```python
from build123d import *


with BuildPart() as f1:
    # F0 (on Top) → F1 (revolve)
    with BuildSketch(Plane.XY):
        with BuildLine():
            Line((5, -24.18787), (5, -20.135133))
            Line((5, -20.135133), (5, -17.787319))
            Line((5, -17.787319), (13, -17.787319))
            Line((13, -17.787319), (25.4, -9.104746))
            Line((25.4, -9.104746), (25.4, 13.497188))
            ThreePointArc((25.4, 13.497188), (24.003098, 16.599398), (20.846833, 17.869453))
            Line((20.846833, 17.869453), (0, 17.869453))
            Line((0, 17.869453), (-20.847, 17.869453))
            ThreePointArc((-20.847, 17.869453), (-24.003206, 16.599388), (-25.4, 13.497184))
            Line((-25.4, 13.497184), (-25.4, -9.104746))
            Line((-25.4, -9.104746), (-13, -17.787319))
            Line((-13, -17.787319), (-5, -17.787319))
            Line((-5, -17.787319), (-5, -20.135133))
            Line((-5, -20.135133), (-5, -24.18787))
            Line((-5, -24.18787), (5, -24.18787))
        make_face()
    revolve(axis=Axis((1.997764, -32.846637, 0), (1, 0, 0)))

    # F2: F1 across plane


with BuildPart() as f1_1:
    add(f1.part)
    add(f1.part.mirror(Plane.XY))


solid = f1_1.part
```
Work out the finished part from the listing and answer in its coordinate system (mm). A direction names the side the tool comes from. Give positions to 0.01 mm unless a question says otherwise; leave off trailing zeros. Loops run counter-clockwise (first coordinate to the right, second up) from the corner with the lowest first, then second, coordinate; pieces in that order, holes last. Notation, with made-up numbers: M 61,19.25 L 76,19.25 A24 ccw 76,48.25 Z; hole C 12.5,21.5 d6. An arc over 180 degrees is marked long. One line per item, written item: value. Start each with the question number.
1. Find section A-A (z = 0). Give the vertices of the cut face in (x, y).
2. Determine the mould class of faces 1 (the face through (-0.292, -39.449, 50.285)), 2 (the face through (-8.944, -18.936, -5.768)), 3 (the face through (-25.4, -54.09, 10.95)) for opening direction Y: released by +Y, released by -Y, zero draft, split by the parting line, or undercut.
3. Which of the six approach directions +Z, -Z, +X, -X, +Y, -Y give full straight-line access (tool end or side, diameter ignored) to faces 4 (the face through (9.056, -18.936, -5.768)), 5 (the face through (25.4, -11.6, 10.95)), 6 (the face through (-5, -26, -6))?
4. Find the intervals of material crossed by probe 1 along X at (y, z) = (-58, 39); probe 2 along Z at (x, y) = (-22, -21); probe 3 along Z at (x, y) = (16.5, -31), in increasing order.
5. Each of these flat-tipped pins is pushed along its axis until it touches: P1, Ø24, axis at y = -31, z = 0.5, coming from the +X side; P2, Ø12, axis at x = -6.5, z = -35, coming from the +Y side; P3, Ø4, axis at x = -6.5, y = -52, coming from the -Z side. Where does it stop, or does it pass through?
6. Find section C-C (x = 15). Give the vertices of the cut face in (y, z).
7. Find section B-B (x = 6.5). Give the vertices of the cut face in (y, z), and give its area (3 significant figures).
Reported:
1. outline: M -25.4,-79.19 A4.56 ccw -20.85,-83.56 L 20.85,-83.56 A4.56 ccw 25.4,-79.19 L 25.4,-56.59 L 13,-47.91 L 5,-47.91 L 5,-41.51 L -5,-41.51 L -5,-47.91 L -13,-47.91 L -25.4,-56.59 Z; M -25.4,-9.1 L -13,-17.79 L -5,-17.79 L -5,-24.19 L 5,-24.19 L 5,-17.79 L 13,-17.79 L 25.4,-9.1 L 25.4,13.5 A4.56 ccw 20.85,17.87 L -20.85,17.87 A4.56 ccw -25.4,13.5 Z
2. face 1: split by the parting line
2. face 2: undercut
2. face 3: zero draft
3. face 4: +X
3. face 5: +Z, -Z, +X, +Y, -Y
3. face 6: -X
4. probe 1: x = -25.4 to 25.4
4. probe 2: z = -49.16 to -17.78, 17.78 to 49.16
4. probe 3: z = -50.68 to -17.41, 17.41 to 50.68
5. P1: stops at x = 5
5. P2: stops at y = 8.76
5. P3: stops at z = -47.73
6. outline: C -32.85,0 d101.43; hole C -32.85,0 d32.92
7. outline: C -32.85,0 d101.43; hole C -32.85,0 d30.12
7. area: 7,370 mm²
